Input: dimensioned drawing with shaded views. Units: mm. Origin: part minimum x, y, z. A direction names the side the tool comes from. Round coordinates to 2 decimals unless told otherwise and drop trailing zeros. Loops run counter-clockwise (first coordinate to the right, second up) from the corner with the lowest first, then second, coordinate; pieces in that order, holes last. Notation, with made-up numbers: (74, 36.25) -> (114, 36.25) arc R18 ccw to (114, 62.25) -> close; hole circle Ø1 at (-7.5, 3). An arc over 180 degrees is marked (long way). Answer as a JSON object with one key per item and string values.
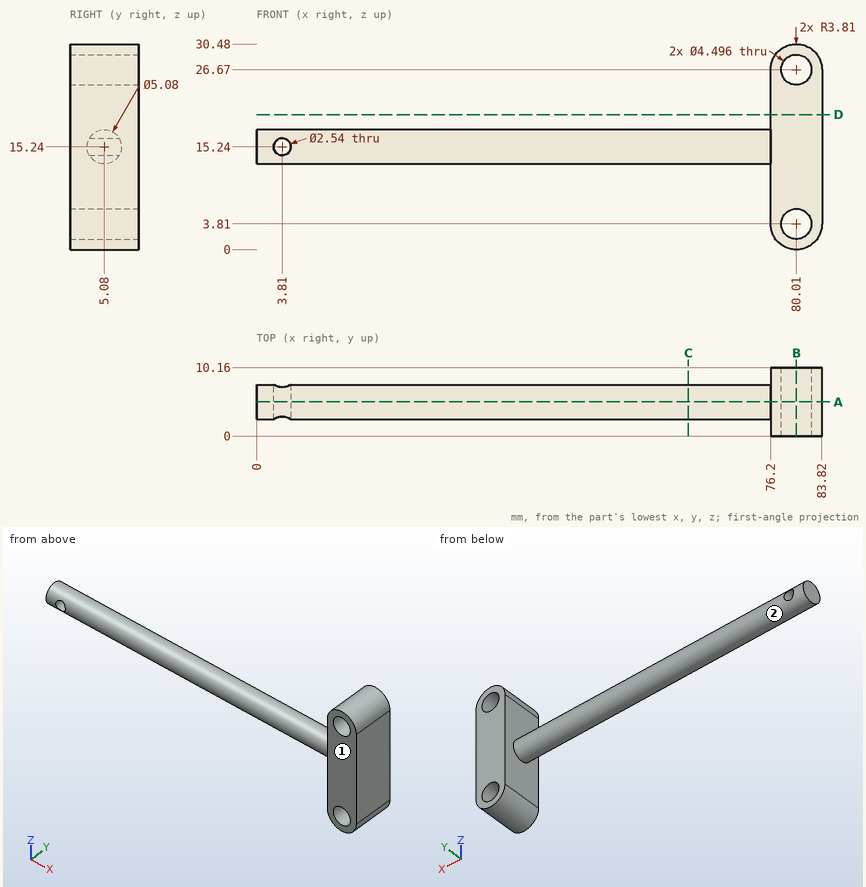
1) Reachability of the marked faces 1 and 2 from +Z, -Z, +X, -X, +Y, -Y: full face, straight path, thin tool, end or side. Return the list, or none.
Output:
{"face 1": "+Z, -Z, +X, -X, -Y", "face 2": "-X"}
2) Section A-A, the plane y = 5.08. Output: boundary loops of the cut face in (x, z), plus the area to 3 significant figures.
Output:
{"outline": "(0, 12.7) -> (76.2, 12.7) -> (76.2, 3.81) arc R3.81 ccw to (83.82, 3.81) -> (83.82, 26.67) arc R3.81 ccw to (76.2, 26.67) -> (76.2, 17.78) -> (0, 17.78) -> close; hole circle Ø2.54 at (3.81, 15.24); hole circle Ø4.5 at (80.01, 3.81); hole circle Ø4.5 at (80.01, 26.67)", "area": "570 mm^2"}
3) Section C-C, the plane x = 64. Output: boundary loops of the cut face in (y, z).
Output:
{"outline": "circle Ø5.08 at (5.08, 15.24)"}
4) Section D-D, the plane z = 20. Output: boundary loops of the cut face in (x, y).
Output:
{"outline": "(76.2, 0) -> (83.82, 0) -> (83.82, 10.16) -> (76.2, 10.16) -> close"}
5) Section B-B, the plane x = 80.01. Output: boundary loops of the cut face in (y, z).
Output:
{"outline": "(0, 0) -> (10.16, 0) -> (10.16, 1.56) -> (0, 1.56) -> close; (0, 6.06) -> (10.16, 6.06) -> (10.16, 24.42) -> (0, 24.42) -> close; (0, 28.92) -> (10.16, 28.92) -> (10.16, 30.48) -> (0, 30.48) -> close"}
6) Ray query, probe 1 along Z at (x, y) = (80.01, 4.75); probe 2 along X at (y, z) = (3.5, 26.67); probe 3 along X at (y, z) = (8.25, 2). Return the intervals inside material, ascending.
Output:
{"probe 1": "z = 0 to 1.56, 6.06 to 24.42, 28.92 to 30.48", "probe 2": "x = 76.2 to 77.76, 82.26 to 83.82", "probe 3": "x = 76.66 to 78.68, 81.34 to 83.36"}
7) Contact query for flat-ended pins moving along their axis: P1, Ø4, axis at x = 42.5, z = 15.5, coming from the +Y side; P2, Ø10, axis at x = 14.5, z = 4, coming from the +Y side; P3, Ø3, axis at y = 7, z = 19.5, coming from the -X side; P4, Ø1, axis at x = 22.5, y = 3.5, coming from the +Z side. Output: stop coordinate, or through.
Output:
{"P1": "stops at y = 7.62", "P2": "passes through", "P3": "stops at x = 76.2", "P4": "stops at z = 17.54"}
